Here's how the part is built. I have some questions about the finished solid (model axes, mm). A direction names the side the tool comes from. Round coordinates to 2 decimals unless told otherwise and drop trailing zeros. Order: outer loops, then holes, each group sorted by start corner. A loop starts at its lowest first (then second) coordinate and runs counter-clockwise, first axis right, second up. Notation, with made-up numbers: (51, -14) -> (83, -14) arc R24 cw to (83, 16) -> close; hole circle Ø9 at (-16, 49.25). An arc over 180 degrees is marked (long way). Answer in a Markdown table with one row per item.
```python
from build123d import *

# Parameters (mm, degrees)
SKETCH1_W           = 60
SKETCH1_H           = 40
BOSS_EXTRUDE1_DEPTH = 60
SKETCH2_W           = 40.5
SKETCH2_H           = 20
CUT_EXTRUDE1_DEPTH  = 39
SKETCH3_R           = 2
CUT_EXTRUDE2_DEPTH  = 5


with BuildPart() as part:
    # Sketch1 → Boss-Extrude1 (new body)
    with BuildSketch(Plane.XY):
        Rectangle(SKETCH1_W, SKETCH1_H)
    extrude(amount=BOSS_EXTRUDE1_DEPTH)

    # Sketch2 → Cut-Extrude1 (cut)
    with BuildSketch(Plane(origin=(0, 0, 0), x_dir=(-1, 0, 0), z_dir=(0, 0, -1))):
        Rectangle(SKETCH2_W, SKETCH2_H)
    extrude(amount=-CUT_EXTRUDE1_DEPTH, mode=Mode.SUBTRACT)

    # Sketch3 → Cut-Extrude2 (cut)
    with BuildSketch(Plane(origin=(0, 0, 0), x_dir=(-1, 0, 0), z_dir=(0, 0, -1))):
        with Locations((26, 17.333333333)):
            Circle(SKETCH3_R)
        with Locations(Location((-26, 17.333333333, 0), (0, 0, 180))):
            Circle(SKETCH3_R)
        with Locations(Location((26, -17.333333333, 0), (0, 0, 180))):
            Circle(SKETCH3_R)
        with Locations((-26, -17.333333333)):
            Circle(SKETCH3_R)
    extrude(amount=-CUT_EXTRUDE2_DEPTH, mode=Mode.SUBTRACT)


solid = part.part
```
1. Suppose I cut it at A-A on z = 24. Write out the boundary of the cut face in (x, y).
Numbers:
| item | result |
|---|---|
| outline | (-30, -20) -> (30, -20) -> (30, 20) -> (-30, 20) -> close; hole (-20.25, -10) -> (20.25, -10) -> (20.25, 10) -> (-20.25, 10) -> close |
2. We'd pull the mould along X, two halves only. Please class faces 1 (the face through (20.25, 0, 19)), 2 (the face through (0, -20, 30)), 3 (the face through (30, 0, 30)): released by +X, released by -X, zero draft, split by the parting line, or undercut.
Numbers:
| item | result |
|---|---|
| face 1 | undercut |
| face 2 | zero draft |
| face 3 | released by +X |
3. For faces 4 (the face through (0, 0, 39)), 5 (the face through (0, 20, 30)), which set-ups out of +Z, -Z, +X, -X, +Y, -Y let a thin tool reach every point of the face, with its end or its side?
Numbers:
| item | result |
|---|---|
| face 4 | -Z |
| face 5 | +Z, -Z, +X, -X, +Y |
4. For pin 1 Ø2.5 at (x, y) = (26, -17.33) entering from -Z; pin 2 Ø6.5 at (x, y) = (-26, 17.33) entering from -Z; pin 3 Ø10 at (x, y) = (-1.5, 3.5) entering from -Z, each with a flat end and sliding along its axis, tell me the tip position at first contact or that it passes through.
Numbers:
| item | result |
|---|---|
| pin 1 | stops at z = 5 |
| pin 2 | stops at z = 0 |
| pin 3 | stops at z = 39 |
5. Suppose I cut it at D-D on x = 26. Write out the boundary of the cut face in (y, z), then the cut area to 3 significant figures.
Numbers:
| item | result |
|---|---|
| outline | (-20, 0) -> (-19.33, 0) -> (-19.33, 5) -> (-15.33, 5) -> (-15.33, 0) -> (15.33, 0) -> (15.33, 5) -> (19.33, 5) -> (19.33, 0) -> (20, 0) -> (20, 60) -> (-20, 60) -> close |
| area | 2,360 mm2 |
6. Suppose I cut it at B-B on x = 5. Write out the boundary of the cut face in (y, z).
Numbers:
| item | result |
|---|---|
| outline | (-20, 0) -> (-10, 0) -> (-10, 39) -> (10, 39) -> (10, 0) -> (20, 0) -> (20, 60) -> (-20, 60) -> close |
7. Please list where these lines run through material, in increasing order: line 1 along Y through (x, z) = (-26, 1); line 2 along X through (y, z) = (8, 19.5); line 3 along Y through (x, z) = (20, 34.5).
Numbers:
| item | result |
|---|---|
| line 1 | y = -20 to -19.33, -15.33 to 15.33, 19.33 to 20 |
| line 2 | x = -30 to -20.25, 20.25 to 30 |
| line 3 | y = -20 to -10, 10 to 20 |
8. Suppose I cut it at C-C on y = -8. Write out the boundary of the cut face in (x, z), then the cut area to 3 significant figures.
Numbers:
| item | result |
|---|---|
| outline | (-30, 0) -> (-20.25, 0) -> (-20.25, 39) -> (20.25, 39) -> (20.25, 0) -> (30, 0) -> (30, 60) -> (-30, 60) -> close |
| area | 2,020 mm2 |
